```python
from build123d import *

# Parameters (mm, degrees)
SKETCH1_R           = 62.70625
SKETCH1_R_2         = 56.3626
BOSS_EXTRUDE1_DEPTH = 6.35
SKETCH5_W           = 19.05
SKETCH5_H           = 18.832271031
BOSS_EXTRUDE2_DEPTH = 6.35
FILLET1_R           = 5.08
SKETCH11_R          = 3.2639
CUT_EXTRUDE2_DEPTH  = 7.35
SKETCH17_W          = 169.784888888
SKETCH17_H          = 116.987853086
CUT_EXTRUDE3_DEPTH  = 7.35
FILLET2_R           = 6.35
SKETCH18_R          = 2.15265
BOSS_EXTRUDE4_DEPTH = 6.35


with BuildPart() as part:
    # Sketch1 → Boss-Extrude1 (new body)
    with BuildSketch(Plane(origin=(0, 0, 0), x_dir=(1, 0, 0), z_dir=(0, 1, 0))):
        Circle(SKETCH1_R)
        Circle(SKETCH1_R_2, mode=Mode.SUBTRACT)
    extrude(amount=BOSS_EXTRUDE1_DEPTH)

    # Sketch5 → Boss-Extrude2 (add)
    with BuildSketch(Plane(origin=(0, 6.35, 0), x_dir=(1, 0, 0), z_dir=(0, 1, 0))):
        with Locations((0, 69.958864484)):
            Rectangle(SKETCH5_W, SKETCH5_H)
    extrude(amount=-BOSS_EXTRUDE2_DEPTH)

    # Fillet1
    fillet1_edges = [part.edges().sort_by_distance(p)[0] for p in [
        (9.525, 3.175, -61.978610537),
        (-9.525, 3.175, -61.978610537),
        (9.525, 3.175, -79.375),
        (-9.525, 3.175, -79.375),
    ]]
    fillet(fillet1_edges, radius=FILLET1_R)

    # Sketch11 → Cut-Extrude2 (cut, through all)
    with BuildSketch(Plane.XZ):
        with Locations((0, -69.85)):
            Circle(SKETCH11_R)
    extrude(amount=-CUT_EXTRUDE2_DEPTH, mode=Mode.SUBTRACT)

    # Sketch17 → Cut-Extrude3 (cut, through all)
    with BuildSketch(Plane(origin=(0, 6.35, 0), x_dir=(1, 0, 0), z_dir=(0, 1, 0))):
        with Locations((0, -21.181326543)):
            Rectangle(SKETCH17_W, SKETCH17_H)
    extrude(amount=-CUT_EXTRUDE3_DEPTH, mode=Mode.SUBTRACT)

    # Fillet2
    fillet2_edges = [part.edges().sort_by_distance(p)[0] for p in [
        (-42.243491333, 3.175, -37.3126),
        (42.243491333, 3.175, -37.3126),
    ]]
    fillet(fillet2_edges, radius=FILLET2_R)

    # Sketch18 → Boss-Extrude4 (add)
    with BuildSketch(Plane(origin=(0, 6.35, 0), x_dir=(1, 0, 0), z_dir=(0, 1, 0))):
        Polygon((-50.396861711, 37.3126), (-70.416081127, 37.3126), (-70.416081127, 44.9326), (-43.739401531, 44.9326), align=None)
        with Locations((-64.77, 41.1226)):
            Circle(SKETCH18_R, mode=Mode.SUBTRACT)
        Polygon((50.396861711, 37.3126), (43.739401531, 44.9326), (70.416081127, 44.9326), (70.416081127, 37.3126), align=None)
        with Locations((64.77, 41.1226)):
            Circle(SKETCH18_R, mode=Mode.SUBTRACT)
    extrude(amount=-BOSS_EXTRUDE4_DEPTH)


solid = part.part
```
Can you work these out from the model? Positions are in its coordinate system, mm. A direction names the side the tool comes from. Coordinates: 2 decimals unless noted, no trailing zeros. Loops run counter-clockwise (first coordinate to the right, second up) from the corner with the lowest first, then second, coordinate; pieces in that order, holes last.
1) Imagine slicing it at C-C on y = 5.25. State how many separate pieces and enclosed holes the cut face has, plus the area to 3 significant figures.
2) Imagine slicing it at B-B on x = 0. List the corners of the cut face in (y, z) for me (3 decimals).
3) Imagine slicing it at A-A on z = -69.85. List the corners of the cut face in (x, y) for me (3 decimals).
4) For pin 1 (1 mm diameter, centred on x = 8, y = 3.5, fed in from +Z); pin 2 (3 mm diameter, centred on y = 5.5, z = -70, fed in from +X) (3 decimals); pin 3 (1 mm diameter, centred on y = 1, z = -70.5, fed in from -X) (3 decimals), each with a flat end and sliding along its axis, tell me the tip position at first contact or that it passes through.
5) Thinking about a two-plate mould opening in X: for faces 4 (the flat face through (-9.525, 3, -70)), 5 (the cylindrical face through (1.755, 3.131, -67.098)), 6 (the flat face through (0, 3, -79.375)), which applies, pulls with the +X half, pulls with the -X half, needs draft (parallel to the pull), parting line crosses it, or undercut?
6) I need wall thicknesses on probe 1 along Z at (x, y) = (-64.77, 3.5); probe 2 along X at (y, z) = (5.5, -41.5); probe 3 along Z at (x, y) = (-53.5, 4.75). Which ranges of each line are inside material? Lowest first, please.
7) Imagine slicing it at D-D on x = 61. List the corners of the cut face in (y, z) for me, plus the area to 3 significant figures.
8) Which directions (+Z, -Z, +X, -X, +Y, -Y) give clear straight access to the entire face, cutting with the end or side of a thin tool? Please do faces 1 (the flat face through (-57, 3, -44.933)), 2 (the cylindrical face through (-42.51, 3.13, -37.83)), 3 (the flat face through (57, 3, -44.933)).
Completed:
1. separate pieces: 1
1. enclosed holes: 3
1. area: 1,280 mm2
2. outline: (0, -79.375) - (6.35, -79.375) - (6.35, -73.114) - (0, -73.114) - close; (0, -66.586) - (6.35, -66.586) - (6.35, -56.363) - (0, -56.363) - close
3. outline: (-9.525, 0) - (-3.264, 0) - (-3.264, 6.35) - (-9.525, 6.35) - close; (3.264, 0) - (9.525, 0) - (9.525, 6.35) - (3.264, 6.35) - close
4. pin 1: stops at z = -55.72
4. pin 2: stops at x = 9.525
4. pin 3: stops at x = -9.525
5. face 4: pulls with the -X half
5. face 5: undercut
5. face 6: needs draft
6. probe 1: z = -44.93 to -43.28, -38.97 to -37.31
6. probe 2: x = -70.42 to -66.89, -62.65 to -38.14, 38.14 to 62.65, 66.89 to 70.42
6. probe 3: z = -44.93 to -37.31
7. outline: (0, -44.93) - (6.35, -44.93) - (6.35, -37.31) - (0, -37.31) - close
7. area: 48.4 mm2
8. face 1: -Z, -X, +Y, -Y
8. face 2: +Z, +Y, -Y
8. face 3: -Z, +X, +Y, -Y
